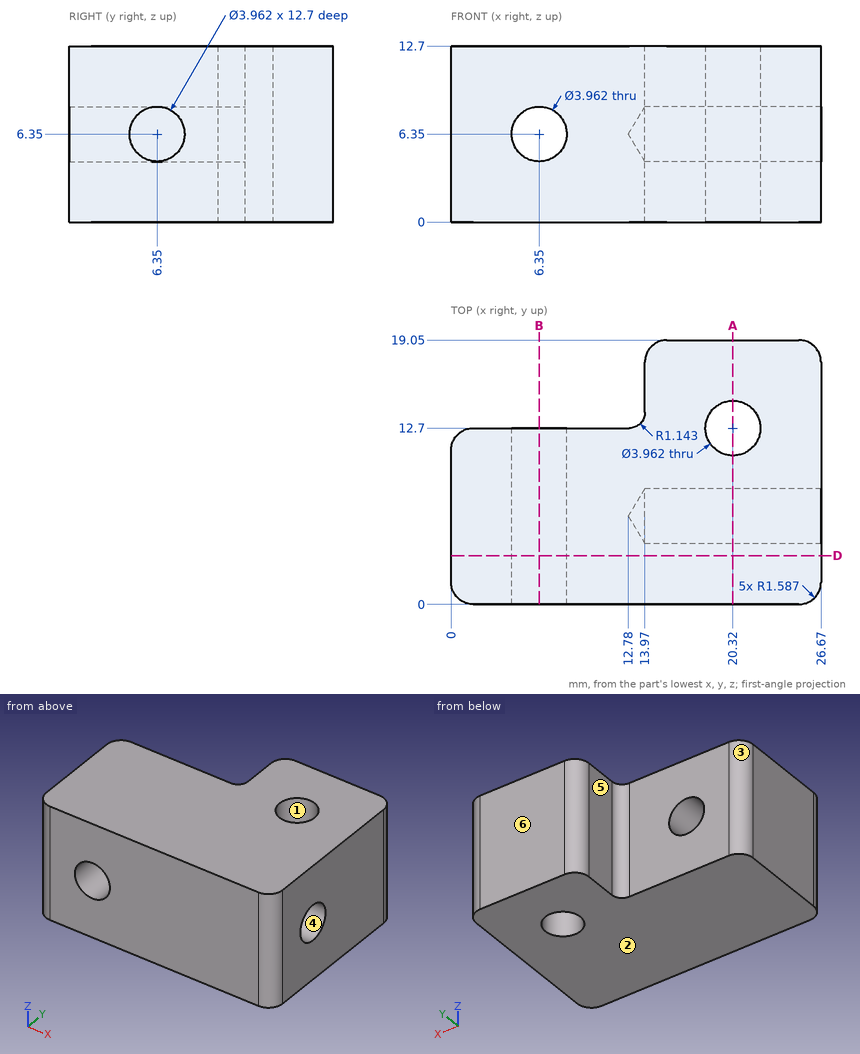
Verification items for this drawing (mm, ordinates from the low corner). A direction names the side the tool comes from. Coordinates: 2 decimals unless noted, no trailing zeros. Order: outer loops, then holes, each group sorted by start corner. A loop starts at its lowest first (then second) coordinate and runs counter-clockwise, first axis right, second up. Notation, with made-up numbers: M 78.25,28 L 131.25,28 A28 cw 131.25,64 Z; hole C -28,28 d7. An arc over 180 degrees is marked long. Use CSV: the item, a comma, the result in double quotes.
Item 1: Gauge pin test, flat ends, axial feed: pin 1 Ø5 at (x, z) = (6.35, 6.35) entering from +Y; pin 2 Ø1.1 at (y, z) = (16, 3.5) entering from -X. Record the tip position at first contact, or that the pin passes through.
Returned:
pin 1,"stops at y = 12.7"
pin 2,"stops at x = 13.97"
Item 2: Thickness scan on line 1 along Z through (x, y) = (6.35, 8.25); line 2 along X through (y, z) = (9, 6.35); line 3 along Y through (x, z) = (20.32, 3). Record the ranges inside material, lowest first.
Returned:
line 1,"z = 0 to 4.37, 8.33 to 12.7"
line 2,"x = 0 to 4.37, 8.33 to 26.67"
line 3,"y = 0 to 10.72, 14.68 to 19.05"
Item 3: Cross-section at D-D on y = 3.5. Record the cut outline in (x, z), then the cut area to 3 significant figures.
Returned:
outline,"M 0,0 L 26.67,0 L 26.67,12.7 L 0,12.7 Z; hole C 6.35,6.35 d3.96"
area,"326 mm2"
Item 4: Cross-section at A-A on x = 20.32. Record the cut outline in (y, z).
Returned:
outline,"M 0,0 L 10.72,0 L 10.72,12.7 L 0,12.7 Z; M 14.68,0 L 19.05,0 L 19.05,12.7 L 14.68,12.7 Z; hole C 6.35,6.35 d3.96"
Item 5: Mould release check, pull along Y, two halves, no side actions. Record for the marked faces 1, 2 and 3: pulls with the +Y half, pulls with the -Y half, needs draft (parallel to the pull), parting line crosses it, or undercut.
Returned:
face 1,"undercut"
face 2,"needs draft"
face 3,"pulls with the +Y half"
Item 6: Tool access check on the marked faces 4, 5 and 6. Record the directions out of +Z, -Z, +X, -X, +Y, -Y that give a thin tool (end or side, any length) a straight path to the whole face; none if there is none.
Returned:
face 4,"+X"
face 5,"+Z, -Z, -X, +Y"
face 6,"+Z, -Z, +X, -X, +Y"
Item 7: Cross-section at B-B on x = 6.35. Record the cut outline in (y, z), then the cut area to 3 significant figures.
Returned:
outline,"M 0,0 L 12.7,0 L 12.7,4.37 L 0,4.37 Z; M 0,8.33 L 12.7,8.33 L 12.7,12.7 L 0,12.7 Z"
area,"111 mm2"
